```python
from build123d import *

# Parameters (mm, degrees)
SKETCH1_R           = 0.5
SKETCH1_R_2         = 1.375
BOSS_EXTRUDE1_DEPTH = 2
SKETCH4_R           = 4.6270037
SKETCH4_R_2         = 2.6270037
BOSS_EXTRUDE3_DEPTH = 2.5
CUT_EXTRUDE3_DEPTH  = 2.5
SKETCH6_R           = 15.875
SKETCH6_R_2         = 3.75
BOSS_EXTRUDE6_DEPTH = 2.54
SKETCH7_R           = 1.778
CUT_EXTRUDE4_DEPTH  = 2.54
CIRPATTERN1_COUNT   = 4


with BuildPart() as part:
    # Sketch1 → Boss-Extrude1 (new body)
    with BuildSketch(Plane(origin=(0, 0, 0), x_dir=(1, 0, 0), z_dir=(0, 1, 0))):
        with BuildLine():
            Line((-4, 4), (-2.467435953, 13.402193757))
            ThreePointArc((-2.467435953, 13.402193757), (0, 15.5), (2.467435953, 13.402193757))
            Line((2.467435953, 13.402193757), (4, 4))
            Line((4, 4), (12.448472752, 2.459445505))
            ThreePointArc((12.448472752, 2.459445505), (14.5, 0), (12.448472752, -2.459445505))
            Line((12.448472752, -2.459445505), (4, -4))
            Line((4, -4), (2.467435953, -13.402193757))
            ThreePointArc((2.467435953, -13.402193757), (0, -15.5), (-2.467435953, -13.402193757))
            Line((-2.467435953, -13.402193757), (-4, -4))
            Line((-4, -4), (-12.448472752, -2.459445505))
            ThreePointArc((-12.448472752, -2.459445505), (-14.5, 0), (-12.448472752, 2.459445505))
            Line((-12.448472752, 2.459445505), (-4, 4))
        make_face()
        with Locations((0, 12)):
            Circle(SKETCH1_R, mode=Mode.SUBTRACT)
        with Locations((0, 9.5)):
            Circle(SKETCH1_R, mode=Mode.SUBTRACT)
        with Locations((0, 7.5)):
            Circle(SKETCH1_R, mode=Mode.SUBTRACT)
        with Locations((12, 0)):
            Circle(SKETCH1_R, mode=Mode.SUBTRACT)
        with Locations((9.5, 0)):
            Circle(SKETCH1_R, mode=Mode.SUBTRACT)
        with Locations((7.5, 0)):
            Circle(SKETCH1_R, mode=Mode.SUBTRACT)
        with Locations((0, -12)):
            Circle(SKETCH1_R, mode=Mode.SUBTRACT)
        with Locations((0, -9.5)):
            Circle(SKETCH1_R, mode=Mode.SUBTRACT)
        with Locations((0, -7.5)):
            Circle(SKETCH1_R, mode=Mode.SUBTRACT)
        with Locations((-12, 0)):
            Circle(SKETCH1_R, mode=Mode.SUBTRACT)
        with Locations((-9.5, 0)):
            Circle(SKETCH1_R, mode=Mode.SUBTRACT)
        with Locations((-7.5, 0)):
            Circle(SKETCH1_R, mode=Mode.SUBTRACT)
        Circle(SKETCH1_R_2, mode=Mode.SUBTRACT)
    extrude(amount=BOSS_EXTRUDE1_DEPTH)

    # Sketch4 → Boss-Extrude3 (add)
    with BuildSketch(Plane.XZ):
        Circle(SKETCH4_R)
        Circle(SKETCH4_R_2, mode=Mode.SUBTRACT)
    extrude(amount=BOSS_EXTRUDE3_DEPTH)

    # Sketch5 → Cut-Extrude3 (cut)
    with BuildSketch(Plane.XZ.offset(2.5)):
        with BuildLine():
            Line((0.282820055, 2.611735296), (0, 3.101594))
            Line((0, 3.101594), (-0.282820055, 2.611735296))
            ThreePointArc((-0.282820055, 2.611735296), (0, 2.6270037), (0.282820055, 2.611735296))
        make_face()
        with BuildLine():
            ThreePointArc((-1.076048447, 2.396511669), (-0.811788788, 2.498428987), (-0.538092735, 2.571304075))
            Line((-0.538092735, 2.571304075), (-0.958445256, 2.949791185))
            Line((-0.958445256, 2.949791185), (-1.076048447, 2.396511669))
        make_face()
        with BuildLine():
            Line((0.958445256, 2.949791185), (0.538092735, 2.571304075))
            ThreePointArc((0.538092735, 2.571304075), (0.811788788, 2.498428987), (1.076048447, 2.396511669))
            Line((1.076048447, 2.396511669), (0.958445256, 2.949791185))
        make_face()
        with BuildLine():
            ThreePointArc((-1.76394572, 1.946700782), (-1.544114033, 2.125290638), (-1.306333259, 2.279175696))
            Line((-1.306333259, 2.279175696), (-1.823071212, 2.509242256))
            Line((-1.823071212, 2.509242256), (-1.76394572, 1.946700782))
        make_face()
        with BuildLine():
            Line((1.823071212, 2.509242256), (1.306333259, 2.279175696))
            ThreePointArc((1.306333259, 2.279175696), (1.544114033, 2.125290638), (1.76394572, 1.946700782))
            Line((1.76394572, 1.946700782), (1.823071212, 2.509242256))
        make_face()
        with BuildLine():
            ThreePointArc((-2.279175696, 1.306333259), (-2.125290638, 1.544114033), (-1.946700782, 1.76394572))
            Line((-1.946700782, 1.76394572), (-2.509242256, 1.823071212))
            Line((-2.509242256, 1.823071212), (-2.279175696, 1.306333259))
        make_face()
        with BuildLine():
            Line((2.509242256, 1.823071212), (1.946700782, 1.76394572))
            ThreePointArc((1.946700782, 1.76394572), (2.125290638, 1.544114033), (2.279175696, 1.306333259))
            Line((2.279175696, 1.306333259), (2.509242256, 1.823071212))
        make_face()
        with BuildLine():
            ThreePointArc((-2.571304075, 0.538092735), (-2.498428987, 0.811788788), (-2.396511669, 1.076048447))
            Line((-2.396511669, 1.076048447), (-2.949791185, 0.958445256))
            Line((-2.949791185, 0.958445256), (-2.571304075, 0.538092735))
        make_face()
        with BuildLine():
            Line((2.949791185, 0.958445256), (2.396511669, 1.076048447))
            ThreePointArc((2.396511669, 1.076048447), (2.498428987, 0.811788788), (2.571304075, 0.538092735))
            Line((2.571304075, 0.538092735), (2.949791185, 0.958445256))
        make_face()
        with BuildLine():
            ThreePointArc((-2.611735296, -0.282820055), (-2.6270037, 0), (-2.611735296, 0.282820055))
            Line((-2.611735296, 0.282820055), (-3.101594, 0))
            Line((-3.101594, 0), (-2.611735296, -0.282820055))
        make_face()
        with BuildLine():
            Line((3.101594, 0), (2.611735296, 0.282820055))
            ThreePointArc((2.611735296, 0.282820055), (2.6270037, 0), (2.611735296, -0.282820055))
            Line((2.611735296, -0.282820055), (3.101594, 0))
        make_face()
        with BuildLine():
            ThreePointArc((-2.396511669, -1.076048447), (-2.498428987, -0.811788788), (-2.571304075, -0.538092735))
            Line((-2.571304075, -0.538092735), (-2.949791185, -0.958445256))
            Line((-2.949791185, -0.958445256), (-2.396511669, -1.076048447))
        make_face()
        with BuildLine():
            Line((2.949791185, -0.958445256), (2.571304075, -0.538092735))
            ThreePointArc((2.571304075, -0.538092735), (2.498428987, -0.811788788), (2.396511669, -1.076048447))
            Line((2.396511669, -1.076048447), (2.949791185, -0.958445256))
        make_face()
        with BuildLine():
            ThreePointArc((-1.946700782, -1.76394572), (-2.125290638, -1.544114033), (-2.279175696, -1.306333259))
            Line((-2.279175696, -1.306333259), (-2.509242256, -1.823071212))
            Line((-2.509242256, -1.823071212), (-1.946700782, -1.76394572))
        make_face()
        with BuildLine():
            Line((2.509242256, -1.823071212), (2.279175696, -1.306333259))
            ThreePointArc((2.279175696, -1.306333259), (2.125290638, -1.544114033), (1.946700782, -1.76394572))
            Line((1.946700782, -1.76394572), (2.509242256, -1.823071212))
        make_face()
        with BuildLine():
            ThreePointArc((-1.306333259, -2.279175696), (-1.544114033, -2.125290638), (-1.76394572, -1.946700782))
            Line((-1.76394572, -1.946700782), (-1.823071212, -2.509242256))
            Line((-1.823071212, -2.509242256), (-1.306333259, -2.279175696))
        make_face()
        with BuildLine():
            Line((1.823071212, -2.509242256), (1.76394572, -1.946700782))
            ThreePointArc((1.76394572, -1.946700782), (1.544114033, -2.125290638), (1.306333259, -2.279175696))
            Line((1.306333259, -2.279175696), (1.823071212, -2.509242256))
        make_face()
        with BuildLine():
            ThreePointArc((-0.538092735, -2.571304075), (-0.811788788, -2.498428987), (-1.076048447, -2.396511669))
            Line((-1.076048447, -2.396511669), (-0.958445256, -2.949791185))
            Line((-0.958445256, -2.949791185), (-0.538092735, -2.571304075))
        make_face()
        with BuildLine():
            Line((0.958445256, -2.949791185), (1.076048447, -2.396511669))
            ThreePointArc((1.076048447, -2.396511669), (0.811788788, -2.498428987), (0.538092735, -2.571304075))
            Line((0.538092735, -2.571304075), (0.958445256, -2.949791185))
        make_face()
        with BuildLine():
            ThreePointArc((0.282820055, -2.611735296), (0, -2.6270037), (-0.282820055, -2.611735296))
            Line((-0.282820055, -2.611735296), (0, -3.101594))
            Line((0, -3.101594), (0.282820055, -2.611735296))
        make_face()
    extrude(amount=-CUT_EXTRUDE3_DEPTH, mode=Mode.SUBTRACT)

    # Sketch6 → Boss-Extrude6 (add)
    with BuildSketch(Plane(origin=(0, 2, 0), x_dir=(1, 0, 0), z_dir=(0, 1, 0))):
        Circle(SKETCH6_R)
        Circle(SKETCH6_R_2, mode=Mode.SUBTRACT)
    extrude(amount=-BOSS_EXTRUDE6_DEPTH)

    # Sketch7 → Cut-Extrude4 (cut)
    with BuildSketch(Plane(origin=(0, 2, 0), x_dir=(1, 0, 0), z_dir=(0, 1, 0))):
        with Locations((0, 9.779)):
            Circle(SKETCH7_R)
    cut_extrude4 = extrude(amount=-CUT_EXTRUDE4_DEPTH, mode=Mode.SUBTRACT)

    # CirPattern1: Cut-Extrude4 ×4 about axis
    cirpattern1_axis = Axis((0, 0, 0), (0, 1, 0))
    for i in range(1, CIRPATTERN1_COUNT):
        add(cut_extrude4.rotate(cirpattern1_axis, i * 360 / CIRPATTERN1_COUNT), mode=Mode.SUBTRACT)


solid = part.part
```
The listing builds one solid part. Answer for the finished solid, in the listing's coordinates (mm). A direction names the side the tool comes from. Give positions to 0.01 mm unless a question says otherwise; leave off trailing zeros. Write each loop counter-clockwise with the first axis right and the second up, starting at its lowest first coordinate (ties: lowest second). Pieces come first, ordered by that corner, then holes. Notation, with made-up numbers: M -12.5,-8.75 L 16.5,-8.75 A27 cw 16.5,16.25 Z; hole C -30.75,15 d7. An arc over 180 degrees is marked long. Write each question's results on one line, items separated by ' | '.
Q1. Section D-D, the plane z = 12.5 is taken. Write down the section's boundary in (x, y), then the cut area to 3 significant figures.
Output values:
outline: M -9.79,-0.54 L 9.79,-0.54 L 9.79,2 L -9.79,2 Z | area: 49.7 mm2
Q2. A tool of negligible diameter and unlimited length cuts with its end or side. For faces 5 (the cylindrical face through (-3.67, -1.51, -2.82)), 6 (the cylindrical face through (0, 1, 8)), from which of +Z, -Z, +X, -X, +Y, -Y can it reach the whole face along a straight path? Write none if from no direction.
Output values:
face 5: -Y | face 6: +Y, -Y
Q3. Section A-A, the plane z = -10.5 is taken. Write down the section's boundary in (x, y), then the cut area to 3 significant figures.
Output values:
outline: M -11.91,-0.54 L -1.63,-0.54 L -1.63,2 L -11.91,2 Z; M 1.63,-0.54 L 11.91,-0.54 L 11.91,2 L 1.63,2 Z | area: 52.2 mm2
Q4. Section B-B, the plane y = 0.6 is taken. Write down the section's boundary in (x, z) (3 decimals), then the cut area to 3 significant figures.
Output values:
outline: C 0,0 d31.75; hole C -9.779,0 d3.556; hole C 0,-9.779 d3.556; hole C 0,9.779 d3.556; hole C 0,0 d2.75; hole C 9.779,0 d3.556 | area: 746 mm2
Q5. Flat-ended cylindrical pins translate along their axes: P1, Ø1.9, axis at x = 1.5, z = 0.5, coming from the -Y side; P2, Ø4, axis at x = 0, z = -9.779, coming from the -Y side; P3, Ø1, axis at x = 3.5, y = 1, coming from the +Z side. Find the tip coordinate at first contact, or state that the pin passes through.
Output values:
P1: y = 0 | P2: y = -0.54 | P3: z = 15.59
Q6. Consider L1, parallel to X at y = 1.45, z = 0 (3 decimals); L2, parallel to Y at x = 2, z = -11. Determine where each line is inside the solid, lowest interval first. Write a range as from..to.
Output values:
L1: -15.875..-11.557, -8.001..-1.375, 1.375..8.001, 11.557..15.875 | L2: -0.54..2
Q7. Section C-C, the plane x = 9 is taken. Write down the section's boundary in (y, z), then the cut area to 3 significant figures.
Output values:
outline: M -0.54,-13.08 L 2,-13.08 L 2,-1.6 L -0.54,-1.6 Z; M -0.54,1.6 L 2,1.6 L 2,13.08 L -0.54,13.08 Z | area: 58.3 mm2
Q8. For a pull along Z with two mould halves and no side action, classify faces 1 (the cylindrical face through (8, 1, 0)), 2 (the flat face through (3, -0.54, -4)), 3 (the cylindrical face through (-3.441, 0.748, 15.497)), 4 (the cylindrical face through (-0.3, 0.99, 1.34)) as released by +Z, released by -Z, zero draft, split by the parting line, or undercut.
Output values:
face 1: undercut | face 2: zero draft | face 3: split by the parting line | face 4: undercut
